from build123d import *

# Parameters (mm, degrees)
BOSS_EXTRUDE1_DEPTH     = 28
SHELL1_T                = -2
CUT_EXTRUDE1_DEPTH      = 12
CUT_EXTRUDE1_DEPTH_BACK = 12
SKETCH9_R               = 6.4
SKETCH12_R              = 4
CUT_EXTRUDE3_DEPTH      = 2
SKETCH17_W              = 36.183766184
SKETCH17_H              = 26
BOSS_EXTRUDE2_DEPTH     = 30
CUT_EXTRUDE14_DEPTH     = 30


with BuildPart() as part:
    # Sketch1 → Boss-Extrude1 (new body)
    with BuildSketch(Plane(origin=(0, 0, 0), x_dir=(1, 0, 0), z_dir=(0, 1, 0))):
        with BuildLine():
            Line((0, 0), (0, 50))
            Line((0, 50), (27, 77))
            Line((27, 77), (77, 77))
            Line((77, 77), (77, 52))
            ThreePointArc((77, 52), (57.56334266, 48.230865133), (40.944353892, 37.46985967))
            Line((40.944353892, 37.46985967), (38.823033548, 39.591180014))
            ThreePointArc((38.823033548, 39.591180014), (33.994606424, 43.005393576), (37.408819986, 38.176966452))
            Line((37.408819986, 38.176966452), (39.53014033, 36.055646108))
            ThreePointArc((39.53014033, 36.055646108), (28.769134867, 19.43665734), (25, 0))
            Line((25, 0), (0, 0))
        make_face()
    extrude(amount=BOSS_EXTRUDE1_DEPTH)

    # Shell1
    shell1_openings = [part.faces().sort_by_distance(p)[0] for p in [
        (57.56334266, 14, -48.230865133),
        (28.769134867, 14, -19.43665734),
    ]]
    offset(amount=SHELL1_T, openings=shell1_openings, kind=Kind.INTERSECTION)

    # Sketch9 → Cut-Extrude1 (cut, two sides: drawn at the far end of the back side and taken through both)
    with BuildSketch(Plane(origin=(0, 14, 0), x_dir=(1, 0, 0), z_dir=(0, 1, 0)).offset(-CUT_EXTRUDE1_DEPTH_BACK)):
        with Locations((36.184678266, 38.815321734)):
            Circle(SKETCH9_R)
    extrude(amount=CUT_EXTRUDE1_DEPTH + CUT_EXTRUDE1_DEPTH_BACK, mode=Mode.SUBTRACT)

    # Sketch12 → Cut-Extrude3 (cut)
    with BuildSketch(Plane(origin=(0, 28, 0), x_dir=(1, 0, 0), z_dir=(0, 1, 0))):
        with Locations(Location((67, 62.5, 0), (0, 0, 270))):
            Circle(SKETCH12_R)
        with Locations(Location((12.5, 10, 0), (0, 0, 270))):
            Circle(SKETCH12_R)
    extrude(amount=-CUT_EXTRUDE3_DEPTH, mode=Mode.SUBTRACT)

    # Sketch17 → Boss-Extrude2 (add)
    with BuildSketch(Plane(origin=(-25, 0, -25), x_dir=(-0.7071067811865435, 0, 0.7071067811865516), z_dir=(-0.7071067811865516, 0, -0.7071067811865435))):
        with Locations((-54.447222151, 14)):
            Rectangle(SKETCH17_W, SKETCH17_H)
    extrude(amount=BOSS_EXTRUDE2_DEPTH)

    # Sketch19_7 → Cut-Extrude14 (cut)
    with BuildSketch(Plane(origin=(0, 27, 0), x_dir=(1, 0, 0), z_dir=(0, 1, 0))):
        with BuildLine():
            Line((-7.176599947, 64.001557861), (3.412478957, 53.412478957))
            Line((3.412478957, 53.412478957), (0.707106781, 50.707106781))
            Line((0.707106781, 50.707106781), (-20.506096654, 71.920310217))
            Line((-20.506096654, 71.920310217), (5.079689783, 97.506096654))
            Line((5.079689783, 97.506096654), (26.292893219, 76.292893219))
            Line((26.292893219, 76.292893219), (5.445665953, 55.445665953))
            Line((5.445665953, 55.445665953), (-5.153515959, 65.947132971))
            ThreePointArc((-5.153515959, 65.947132971), (-8.165921561, 77.734505129), (0.807292373, 85.950231609))
            Line((0.807292373, 85.950231609), (5.671042553, 81.08648143))
            Line((5.671042553, 81.08648143), (4.410448732, 76.512705214))
            Line((4.410448732, 76.512705214), (9.448954094, 81.551210575))
            Line((9.448954094, 81.551210575), (2.047814256, 88.952350413))
            ThreePointArc((2.047814256, 88.952350413), (-10.556487738, 79.431665635), (-7.176599947, 64.001557861))
        make_face()
    extrude(amount=-CUT_EXTRUDE14_DEPTH, mode=Mode.SUBTRACT)


solid = part.part
Design review of the part built by this model. Coordinates are the model's own, in mm. A direction names the side the tool comes from. Give positions to 0.01 mm unless a question says otherwise; leave off trailing zeros. Write each loop counter-clockwise with the first axis right and the second up, starting at its lowest first coordinate (ties: lowest second). Pieces come first, ordered by that corner, then holes. Notation, with made-up numbers: M 43,-38 L 81,-38 A21 cw 81,-24 Z; hole C 73.25,39.25 d4. An arc over 180 degrees is marked long. Answer as a JSON object with one key per item and string values. Group by question number.
1) For line 1 along Y through (x, z) = (21.5, -56); line 2 along Z through (x, y) = (3, 7); line 3 along X through (y, z) = (7.75, -12.5), list the stretches that pass through material, from the lowest coordinate up.
2) Tool access review of faces 1 (the face through (-1.956, 14.182, -58.781)), 2 (the face through (63.451, 27.014, -60.654)), 3 (the face through (14, 14, -2)), 4 (the face through (39.899, 0.986, -38.516)): name each direction out of +Z, -Z, +X, -X, +Y, -Y from which nothing blocks a thin tool from reaching the whole face with its end or side.
3) We need section B-B (x = 67). Give the boundary of the cut face in (y, z), and give its area (3 significant figures).
4) We need section A-A (z = -10). Give the boundary of the cut face in (x, y), and give its area (3 significant figures).
5) Clearance check with flat-ended pins moving along their axes: pin 1 Ø16.5 at (x, z) = (3, -73.5) entering from +Y; pin 2 Ø5.5 at (x, z) = (36.12, -40.88) entering from -Y; pin 3 Ø7 at (y, z) = (19, -62.5) entering from -X; pin 4 Ø11.5 at (x, y) = (14.5, 19) entering from -Z. State where each tip first meets the part, or that it passes through.
6) We need section D-D (y = 20.75). Give the boundary of the cut face in (x, z).
7) We need section C-C (z = -68). Give the boundary of the cut face in (x, y).
8) Mouldability with a two-part tool opening along Y and no side actions: class faces 5 (the face through (30, 28, -48)), 6 (the face through (0.22, 14.182, -60.623)), 7 (the face through (2, 14, -25)) as released by +Y, released by -Y, zero draft, split by the parting line, or undercut.
Answer key:
{
 "1": {"line 1": "y = 0 to 2, 26 to 28", "line 2": "z = -88 to -83.76, -57.87 to -53.82, -53 to -50.17, -2 to 0", "line 3": "x = 0 to 2"},
 "2": {"face 1": "-X, +Y, -Y", "face 2": "+Y", "face 3": "+X", "face 4": "+Y, -Y"},
 "3": {"outline": "M 0,-77 L 28,-77 L 28,-66.5 L 26,-66.5 L 26,-75 L 2,-75 L 2,-51.03 L 0,-51.03 Z; M 26,-58.5 L 28,-58.5 L 28,-51.03 L 26,-51.03 Z", "area": "136 mm²"},
 "4": {"outline": "M 0,0 L 25.97,0 L 25.97,2 L 2,2 L 2,26 L 8.5,26 L 8.5,28 L 0,28 Z; M 16.5,26 L 25.97,26 L 25.97,28 L 16.5,28 Z", "area": "136 mm²"},
 "5": {"pin 1": "stops at y = 27", "pin 2": "passes through", "pin 3": "stops at x = -8.85", "pin 4": "stops at z = -82.25"},
 "6": {"outline": "M -7.18,-64 A14.64 ccw 2.05,-88.95 L 9.45,-81.55 L 4.41,-76.51 L 5.67,-81.09 L 0.81,-85.95 A11.84 cw -5.15,-65.95 L 5.45,-55.45 L 27,-77 L 77,-77 L 77,-52 A52 cw 75,-51.96 L 75,-75 L 27.83,-75 L 2,-49.17 L 2,-2 L 25.04,-2 A52 cw 25,0 L 0,0 L 0,-50 L 3.41,-53.41 Z; M 31.9,-43.57 A5 ccw 40.15,-43.84 A6.4 cw Z"},
 "7": {"outline": "M -10.01,1 L -6.81,1 L -6.81,27 L -10.01,27 Z; M 18,0 L 77,0 L 77,28 L 18,28 Z; hole M 20.83,2 L 75,2 L 75,26 L 20.83,26 Z"},
 "8": {"face 5": "released by +Y", "face 6": "zero draft", "face 7": "undercut"}
}
